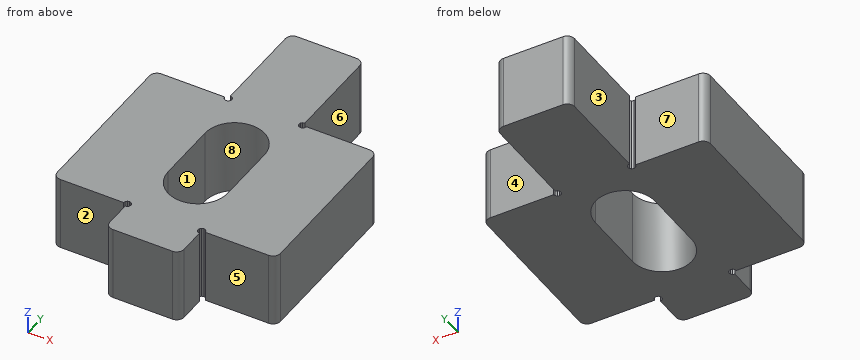
from build123d import *

# Parameters (mm, degrees)
BOSS_EXTRU_1_DEPTH = 5


with BuildPart() as part:
    # Esquisse1 → Boss.-Extru.1 (new body)
    with BuildSketch(Plane.XY.offset(5)):
        with BuildLine():
            Line((10, 14.25), (10, 20.5))
            ThreePointArc((10, 20.5), (9.853553391, 20.853553391), (9.5, 21))
            Line((9.5, 21), (5.5, 21))
            ThreePointArc((5.5, 21), (5.146446609, 20.853553391), (5, 20.5))
            Line((5, 20.5), (5, 14.25))
            Line((5, 14.25), (5.125, 14.21651))
            Line((5.125, 14.21651), (5.216506, 14.125))
            Line((5.216506, 14.125), (5.25, 14))
            Line((5.25, 14), (5.216506, 13.875))
            Line((5.216506, 13.875), (5.125, 13.78349))
            Line((5.125, 13.78349), (5, 13.75))
            Line((5, 13.75), (4.875, 13.78349))
            Line((4.875, 13.78349), (4.783494, 13.875))
            Line((4.783494, 13.875), (4.75, 14))
            Line((4.75, 14), (0.5, 14))
            ThreePointArc((0.5, 14), (0.146446609, 13.853553391), (0, 13.5))
            Line((0, 13.5), (0, 3))
            ThreePointArc((0, 3), (0.146446609, 2.646446609), (0.5, 2.5))
            Line((0.5, 2.5), (4.75, 2.5))
            Line((4.75, 2.5), (4.783494, 2.625))
            Line((4.783494, 2.625), (4.875, 2.716506))
            Line((4.875, 2.716506), (5, 2.75))
            Line((5, 2.75), (5.125, 2.716506))
            Line((5.125, 2.716506), (5.216506, 2.625))
            Line((5.216506, 2.625), (5.25, 2.5))
            Line((5.25, 2.5), (5.216506, 2.375))
            Line((5.216506, 2.375), (5.125, 2.283494))
            Line((5.125, 2.283494), (5, 2.25))
            Line((5, 2.25), (5, 0.4999999))
            ThreePointArc((5, 0.4999999), (5.14644658, 0.14644658), (5.4999999, 0))
            Line((5.4999999, 0), (9.5, 0))
            ThreePointArc((9.5, 0), (9.853553391, 0.146446609), (10, 0.5))
            Line((10, 0.5), (10, 2.25))
            Line((10, 2.25), (9.875, 2.283494))
            Line((9.875, 2.283494), (9.783493, 2.375))
            Line((9.783493, 2.375), (9.75, 2.5))
            Line((9.75, 2.5), (9.783493, 2.625))
            Line((9.783493, 2.625), (9.875, 2.716506))
            Line((9.875, 2.716506), (10, 2.75))
            Line((10, 2.75), (10.125, 2.716506))
            Line((10.125, 2.716506), (10.21651, 2.625))
            Line((10.21651, 2.625), (10.25, 2.5))
            Line((10.25, 2.5), (14.5, 2.5))
            ThreePointArc((14.5, 2.5), (14.853553391, 2.646446609), (15, 3))
            Line((15, 3), (15, 13.5))
            ThreePointArc((15, 13.5), (14.853553391, 13.853553391), (14.5, 14))
            Line((14.5, 14), (10.25, 14))
            Line((10.25, 14), (10.21651, 13.875))
            Line((10.21651, 13.875), (10.125, 13.78349))
            Line((10.125, 13.78349), (10, 13.75))
            Line((10, 13.75), (9.875, 13.78349))
            Line((9.875, 13.78349), (9.783493, 13.875))
            Line((9.783493, 13.875), (9.75, 14))
            Line((9.75, 14), (9.783493, 14.125))
            Line((9.783493, 14.125), (9.875, 14.21651))
            Line((9.875, 14.21651), (10, 14.25))
        make_face()
        with BuildLine():
            Line((5.5, 10.5), (5.5, 6.3))
            ThreePointArc((5.5, 6.3), (7.5, 4.3), (9.5, 6.3))
            Line((9.5, 6.3), (9.5, 10.5))
            ThreePointArc((9.5, 10.5), (7.5, 12.5), (5.5, 10.5))
        make_face(mode=Mode.SUBTRACT)
    extrude(amount=-BOSS_EXTRU_1_DEPTH)


solid = part.part
Can you work these out from the model? Positions are in its coordinate system, mm. Face numbers are marked on the shaded views. A direction names the side the tool comes from. Give positions to 0.01 mm unless a question says otherwise; leave off trailing zeros. Order: outer loops, then holes, each group sorted by start corner. A loop starts at its lowest first (then second) coordinate and runs counter-clockwise, first axis right, second up. Notation, with made-up numbers: M 22.25,78.25 L 34.25,78.25 A18 ccw 34.25,91.25 Z; hole C 50.25,2.25 d4. An arc over 180 degrees is marked long. Use a Markdown table: item, result. Add a question column.
Item 1: Suppose I cut it at C-C (x = 2.75). List the corners of the cut face in (y, z) for me, then the cut area to 3 significant figures.
Item 2: We'd pull the mould along Y, two halves only. Please class the marked faces 1, 2, 3 and 4: +Y half, -Y half, draft (parallel to the pull), parting line (faces both ways), or undercut.
Item 3: For the marked faces 5, 6, 7 and 8, which set-ups out of +Z, -Z, +X, -X, +Y, -Y let a thin tool reach every point of the face, with its end or its side?
Item 4: Suppose I cut it at B-B (x = 7.5). List the corners of the cut face in (y, z) for me, then the cut area to 3 significant figures.
Item 5: Suppose I cut it at D-D (y = 17). List the corners of the cut face in (x, z) for me.
Item 6: Will these pins go through, and if not, where does the flat tip stop? pin 1 (1.5 mm diameter, centred on x = 12.5, z = 3.5, fed in from -Y); pin 2 (0.5 mm diameter, centred on y = 1, z = 2, fed in from -X); pin 3 (0.5 mm diameter, centred on y = 1.5, z = 3.5, fed in from +X).
Item 7: Suppose I cut it at A-A (y = 9). List the corners of the cut face in (x, z) for me, then the cut area to 3 significant figures.
Item 8: If I drill on L1, parallel to X at y = 6.75, z = 0.3; L2, parallel to Y at x = 1.25, z = 1.7; L3, parallel to X at y = 5.5, z = 2.4, over which ranges is the centre line in solid material (lowest first)? Write a range as [from, to].
Answer sheet:
| question | item | result |
|---|---|---|
| 1 | outline | M 2.5,0 L 14,0 L 14,5 L 2.5,5 Z |
| 1 | area | 57.5 mm² |
| 2 | face 1 | undercut |
| 2 | face 2 | -Y half |
| 2 | face 3 | draft |
| 2 | face 4 | +Y half |
| 3 | face 5 | +Z, -Z, +X, -Y |
| 3 | face 6 | +Z, -Z, +X, +Y |
| 3 | face 7 | +Z, -Z, -X, +Y |
| 3 | face 8 | +Z, -Z |
| 4 | outline | M 0,0 L 4.3,0 L 4.3,5 L 0,5 Z; M 12.5,0 L 21,0 L 21,5 L 12.5,5 Z |
| 4 | area | 64.0 mm² |
| 5 | outline | M 5,0 L 10,0 L 10,5 L 5,5 Z |
| 6 | pin 1 | stops at y = 2.5 |
| 6 | pin 2 | stops at x = 5 |
| 6 | pin 3 | stops at x = 10 |
| 7 | outline | M 0,0 L 5.5,0 L 5.5,5 L 0,5 Z; M 9.5,0 L 15,0 L 15,5 L 9.5,5 Z |
| 7 | area | 55.0 mm² |
| 8 | L1 | x = [0, 5.5], [9.5, 15] |
| 8 | L2 | y = [2.5, 14] |
| 8 | L3 | x = [0, 5.67], [9.33, 15] |
